```python
from build123d import *

# Parameters (mm, degrees)
SKETCH_3_R          = 3
EXTRUDE_1_DEPTH     = 3
FILLET_1_R          = 200
FILLET_3_R          = 50
SKETCH_4_R          = 1.25
CUT_EXTRUDE_1_DEPTH = 133.803621182
SKETCH_4_3_R        = 2
SKETCH_4_3_R_2      = 1.25
CUT_EXTRUDE_2_DEPTH = 1.5
FILLET_4_R          = 10
FILLET_5_R          = 10
FILLET_6_R          = 100


# Some blends are built 0.0001 mm under size
with BuildPart() as part:
    # 草图3 → 凸台-拉伸1 (new body)
    with BuildSketch(Plane(origin=(0, 0, 0), x_dir=(1, 0, 0), z_dir=(0, 1, 0))):
        with BuildLine():
            ThreePointArc((3.438749824, 0), (-1, 3.55), (-5.438749824, 0))
            Line((-5.438749824, 0), (-20, 0))
            Line((-20, 0), (-58.823128982, -31.75206117))
            Line((-58.823128982, -31.75206117), (-90.575190152, -70.575190152))
            ThreePointArc((-90.575190152, -70.575190152), (-90.944000004, -79.022324522), (-82.561153427, -80.12594721))
            Line((-82.561153427, -80.12594721), (-53.071679833, -59.477195502))
            Line((-53.071679833, -59.477195502), (-58.807444196, -51.285675059))
            Line((-58.807444196, -51.285675059), (-45.701011487, -42.108452077))
            Line((-45.701011487, -42.108452077), (-39.965247124, -50.29997252))
            Line((-39.965247124, -50.29997252), (0, -22.316005218))
            Line((0, -22.316005218), (100.609346717, -9.962730758))
            ThreePointArc((100.609346717, -9.962730758), (104.990673992, -4.694757302), (100, 0))
            Line((100, 0), (3.438749824, 0))
        make_face()
        with BuildLine():
            Line((0.2, -0.018929156), (0.2, -1.981070844))
            ThreePointArc((0.2, -1.981070844), (-2.55, -1), (0.2, -0.018929156))
        make_face(mode=Mode.SUBTRACT)
        with BuildLine():
            ThreePointArc((-19.8, -16.981070844), (-22.55, -16), (-19.8, -15.018929156))
            Line((-19.8, -15.018929156), (-19.8, -16.981070844))
        make_face(mode=Mode.SUBTRACT)
        with BuildLine():
            ThreePointArc((101.2, -5.981070844), (98.45, -5), (101.2, -4.018929156))
            Line((101.2, -4.018929156), (101.2, -5.981070844))
        make_face(mode=Mode.SUBTRACT)
        with Locations(Location((-86.150380304, -75, 0), (0, 0, 270))):
            Circle(SKETCH_3_R, mode=Mode.SUBTRACT)
    extrude(amount=EXTRUDE_1_DEPTH)

    # 圆角1
    # the kernel refuses this fillet: 200 mm, written as the material it adds along each edge
    with BuildSketch(Plane(origin=(0, 0, 22.316005218), x_dir=(-0.8191520442889868, 0, 0.5735764363510532), z_dir=(0, 1, 0))) as fillet_1_piece_1:
        with BuildLine():
            CenterArc((49.871110762, 199.997070178), FILLET_1_R, 242, 27.689869999)
            Line((-44.023201795, 23.407551606), (-45.901088046, 19.875761235))
            Line((-45.901088046, 19.875761235), (-1.877886251, -3.531790371))
            Line((-1.877886251, -3.531790371), (0, -4))
            ThreePointArc((0, -4), (24.394279061, -4), (48.76690707, -3.999941404))
            Line((48.76690707, -3.999941404), (48.788558122, 0))
        make_face()
    extrude(amount=3)

    # 圆角3
    # the kernel refuses this fillet: 50 mm, written as the material it adds along each edge
    with BuildSketch(Plane(origin=(3.438749824, 0, 0), x_dir=(-0.6554771924780477, 0, -0.7552149694895463), z_dir=(0, 1, 0))) as fillet_3_piece_1:
        with BuildLine():
            CenterArc((27.982022488, -44.040522037), FILLET_3_R, 118.259718548, 20.784438328)
            Line((-9.778725986, -11.266662413), (-10.533940956, -10.611185221))
            Line((-10.533940956, -10.611185221), (-0.755214969, 0.655477192))
            Line((-0.755214969, 0.655477192), (0.473469078, 0.880810441))
            ThreePointArc((0.473469078, 0.880810441), (2.154284303, 0.457687505), (3.835099529, 0.880810441))
            Line((3.835099529, 0.880810441), (4.308568607, 0))
        make_face()
    extrude(amount=3)
    with BuildSketch(Plane(origin=(-5.438749824, 0, 0), x_dir=(-1, 0, 0), z_dir=(0, 1, 0))) as fillet_3_piece_2:
        with BuildLine():
            CenterArc((14.921910743, -49.998699223), FILLET_3_R, 90.413290151, 20.374998027)
            Line((-2.823882627, -3.253787011), (-3.178798495, -2.318888767))
            ThreePointArc((-3.178798495, -2.318888767), (-1.757658507, -1.32685396), (-0.975549412, 0.21978022))
            Line((-0.975549412, 0.21978022), (0, 1))
            ThreePointArc((0, 1), (7.280625088, 1), (14.554036965, 0.999973984))
            Line((14.554036965, 0.999973984), (14.561250176, 0))
        make_face()
    extrude(amount=3)

    # 草图4 → 切除-拉伸1 (cut, through all)
    with BuildSketch(Plane(origin=(0, 3, 0), x_dir=(1, 0, 0), z_dir=(0, 1, 0))):
        with Locations(Location((70.2, -9, 0), (0, 0, 270))):
            Circle(SKETCH_4_R)
        with Locations(Location((0, -20, 0), (0, 0, 270))):
            Circle(SKETCH_4_R)
        with Locations(Location((-45, -30, 0), (0, 0, 270))):
            Circle(SKETCH_4_R)
        with Locations(Location((-15, -8, 0), (0, 0, 270))):
            Circle(SKETCH_4_R)
    extrude(amount=-CUT_EXTRUDE_1_DEPTH, mode=Mode.SUBTRACT)

    # 草图4<3> → 切除-拉伸2 (cut)
    # profile 1 of 4: a face of its own
    with BuildSketch(Plane(origin=(0, 3, 0), x_dir=(1, 0, 0), z_dir=(0, 1, 0))):
        with Locations(Location((70.2, -9, 0), (0, 0, 270))):
            Circle(SKETCH_4_3_R)
        with Locations(Location((70.2, -9, 0), (0, 0, 270))):
            Circle(SKETCH_4_3_R_2, mode=Mode.SUBTRACT)
    # profile 2 of 4: a face of its own
    with BuildSketch(Plane(origin=(0, 3, 0), x_dir=(1, 0, 0), z_dir=(0, 1, 0))):
        with Locations(Location((0, -20, 0), (0, 0, 270))):
            Circle(SKETCH_4_3_R)
        with Locations(Location((0, -20, 0), (0, 0, 270))):
            Circle(SKETCH_4_3_R_2, mode=Mode.SUBTRACT)
    # profile 3 of 4: a face of its own
    with BuildSketch(Plane(origin=(0, 3, 0), x_dir=(1, 0, 0), z_dir=(0, 1, 0))):
        with Locations(Location((-45, -30, 0), (0, 0, 270))):
            Circle(SKETCH_4_3_R)
        with Locations(Location((-45, -30, 0), (0, 0, 270))):
            Circle(SKETCH_4_3_R_2, mode=Mode.SUBTRACT)
    # profile 4 of 4: a face of its own
    with BuildSketch(Plane(origin=(0, 3, 0), x_dir=(1, 0, 0), z_dir=(0, 1, 0))):
        with Locations(Location((-15, -8, 0), (0, 0, 270))):
            Circle(SKETCH_4_3_R)
        with Locations(Location((-15, -8, 0), (0, 0, 270))):
            Circle(SKETCH_4_3_R_2, mode=Mode.SUBTRACT)
    extrude(amount=-CUT_EXTRUDE_2_DEPTH, mode=Mode.SUBTRACT)

    # 圆角4
    fillet_4_edges = [part.edges().sort_by_distance(p)[0] for p in [
        (-53.071679833, 1.5, 59.477195502),
    ]]
    fillet(fillet_4_edges, radius=FILLET_4_R - 0.0001)  # a hair under: the kernel refuses the full size

    # 圆角5
    # the kernel refuses this fillet: 10 mm, written as the material it adds along each edge
    with BuildSketch(Plane(origin=(-45.701011487, 0, 42.108452077), x_dir=(-0.8191520442889864, 0, 0.5735764363510539), z_dir=(0, 1, 0))) as fillet_5_piece_1:
        with BuildLine():
            CenterArc((FILLET_5_R, FILLET_5_R), FILLET_5_R, 180, 90)
            Line((0, FILLET_5_R), (0, 0))
            Line((0, 0), (FILLET_5_R, 0))
        make_face()
    extrude(amount=3)
    with BuildSketch(Plane(origin=(-58.807444196, 0, 51.285675059), x_dir=(0.3420261980761126, 0, 0.9396904170148804), z_dir=(0, 1, 0))) as fillet_5_piece_2:
        with BuildLine():
            CenterArc((7.764622652, 9.659249058), FILLET_5_R, 194.999630824, 60.000165399)
            Line((-1.894652287, 7.071120845), (-2.860579781, 6.812308023))
            Line((-2.860579781, 6.812308023), (-0.965927494, -0.258812821))
            Line((-0.965927494, -0.258812821), (0.258812821, -0.965927494))
            ThreePointArc((0.258812821, -0.965927494), (0.258909414, -0.965901613), (4.917575367, -0.965924906))
            Line((4.917575367, -0.965924906), (5.176397847, 0))
        make_face()
    extrude(amount=3)

    # 圆角6
    fillet_6_edges = [part.edges().sort_by_distance(p)[0] for p in [
        (-58.823128982, 1.5, 31.75206117),
        (-20, 1.5, 0),
    ]]
    fillet(fillet_6_edges, radius=FILLET_6_R)


solid = part.part
```
Model file for the job. Use its own axes, mm. A direction names the side the tool comes from. Coordinates: 2 decimals unless noted, no trailing zeros. Order: outer loops, then holes, each group sorted by start corner. A loop starts at its lowest first (then second) coordinate and runs counter-clockwise, first axis right, second up. Notation, with made-up numbers: (79.5, -8.5) -> (91.5, -8.5) arc R28 ccw to (91.5, 12.5) -> close; hole circle Ø2 at (71, 78.25). An arc over 180 degrees is marked (long way). Answer as a JSON object with one key per item and string values. Group by question number.
1) Cut at B-B, the plane x = 53.5. Write the cut outline in (y, z).
2) Flat gauge pins, fed straight in: pin 1 (4 mm diameter, centred on x = 70.2, z = 9, fed in from -Y); pin 2 (1.5 mm diameter, centred on y = 2.5, z = 8.5, fed in from +X); pin 3 (1 mm diameter, centred on y = 1.5, z = 16, fed in from -X); pin 4 (2 mm diameter, centred on x = -14.5, z = 7.5, fed in from +Y). Where does each tip first touch, or does it go through?
3) Which spindle directions (+Z, -Z, +X, -X, +Y, -Y) get a long thin tool onto all of the face, cutting with end or side? Do faces 1 (the face through (-45.2, 1.48, 20.61)), 2 (the face through (-1.2, 2.3, 18.4)). Say none if no direction does.
4) Drill centre lines: L1, parallel to X at y = 1.1, z = 1; L2, parallel to X at y = 2.2, z = 30; L3, parallel to Z at x = -65, y = 2.2. Where is each one in solid material? Low to high.
5) Pull direction Z, two halves, no side cores. Call faces 3 (the face through (-46.774, 2.26, 30.923)), 4 (the face through (-7, 3, 22)), 5 (the face through (1, 1.5, 21)), 6 (the face through (-23.2, 1.52, 5.09)): +Z half, -Z half, draft (parallel to the pull), parting line (faces both ways), or undercut.
6) Cut at C-C, the plane z = 58.5. Write the cut outline in (x, y).
7) Cut at A-A, the plane y = 2.15. Count the separate pieces of the cut face and the enclosed holes in it, then the cut area to 3 significant figures.
Check values:
{
 "1": {"outline": "(0, 0) -> (3, 0) -> (3, 15.75) -> (0, 15.75) -> close"},
 "2": {"pin 1": "stops at y = 0", "pin 2": "stops at x = 104.18", "pin 3": "stops at x = -40.17", "pin 4": "stops at y = 1.5"},
 "3": {"face 1": "-Z, -X, +Y, -Y", "face 2": "+Y"},
 "4": {"L1": "x = -14.55 to -2.55, 0.2 to 103", "L2": "x = -56.3 to -47, -43 to -2.74", "L3": "z = 39.31 to 67.83"},
 "5": {"face 3": "undercut", "face 4": "draft", "face 5": "undercut", "face 6": "-Z half"},
 "6": {"outline": "(-80.7, 0) -> (-57.11, 0) -> (-57.11, 3) -> (-80.7, 3) -> close"},
 "7": {"separate pieces": "1", "enclosed holes": "8", "area": "4,260 mm²"}
}
